Design review of the part built by this model. Coordinates are the model's own, in mm. A direction names the side the tool comes from. Give positions to 0.01 mm unless a question says otherwise; leave off trailing zeros. Order: outer loops, then holes, each group sorted by start corner. A loop starts at its lowest first (then second) coordinate and runs counter-clockwise, first axis right, second up. Notation, with made-up numbers: (32.25, 8.5) -> (74.25, 8.5) arc R21 ccw to (74.25, 13.5) -> close; hole circle Ø2 at (27, 12). An arc over 180 degrees is marked (long way). Return JSON: item names as keys, results as strings.
```python
from build123d import *

# Parameters (mm, degrees)
ESBO_O2_W                  = 2.6
ESBO_O2_H                  = 5.7
CORTE_EXTRUS_O1_DEPTH      = 8
CORTE_EXTRUS_O2_START      = -20
ESBO_O2_2_W                = 2.6
ESBO_O2_2_H                = 5.7
CORTE_EXTRUS_O2_DEPTH      = 8
CORTE_EXTRUS_O3_DEPTH      = 27.223844112
CORTE_EXTRUS_O3_DEPTH_BACK = 27.223844112
ESBO_O3_R                  = 1.65


with BuildPart() as part:
    # Esboço1 → Revolução1 (revolve)
    with BuildSketch(Plane.XY, mode=Mode.PRIVATE) as revolu_o1_sk:
        Polygon((3.05, 20), (10, 20), (10, 0), (2.4, 0), (2.4, 8), (3.05, 8), align=None)
    revolve(revolu_o1_sk.sketch.rotate(Axis((0, 0, 0), (0, 1, 0)), 90), axis=Axis((0, 0, 0), (0, 1, 0)))

    # Esboço2 → Corte-extrusão1 (cut)
    with BuildSketch(Plane(origin=(0, 20, 0), x_dir=(1, 0, 0), z_dir=(0, 1, 0))):
        with Locations((5, 0)):
            Rectangle(ESBO_O2_W, ESBO_O2_H)
        with Locations((-5, 0)):
            Rectangle(ESBO_O2_W, ESBO_O2_H)
    extrude(amount=-CORTE_EXTRUS_O1_DEPTH, mode=Mode.SUBTRACT)

    # Esboço2<2> → Corte-extrusão2 (cut)
    with BuildSketch(Plane(origin=(0, 20, 0), x_dir=(1, 0, 0), z_dir=(0, 1, 0)).offset(CORTE_EXTRUS_O2_START)):
        with Locations((5, 0)):
            Rectangle(ESBO_O2_2_W, ESBO_O2_2_H)
        with Locations((-5, 0)):
            Rectangle(ESBO_O2_2_W, ESBO_O2_2_H)
    extrude(amount=CORTE_EXTRUS_O2_DEPTH, mode=Mode.SUBTRACT)

    # Esboço3 → Corte-extrusão3 (cut, two sides: drawn at the far end of the back side and taken through both)
    with BuildSketch(Plane.ZY.offset(3.7).offset(-CORTE_EXTRUS_O3_DEPTH_BACK)):
        with Locations((0, 4)):
            Circle(ESBO_O3_R)
        with Locations((0, 16)):
            Circle(ESBO_O3_R)
    extrude(amount=CORTE_EXTRUS_O3_DEPTH + CORTE_EXTRUS_O3_DEPTH_BACK, mode=Mode.SUBTRACT)


solid = part.part
```
Item 1: For pin 1 (2 mm diameter, centred on y = 13, z = -3, fed in from -X); pin 2 (3 mm diameter, centred on x = 5, y = 12.5, fed in from -Z); pin 3 (1.3 mm diameter, centred on x = 5, y = 15, fed in from -Z); pin 4 (2.5 mm diameter, centred on y = 4, z = 0, fed in from +X), all flat-tipped, find the tip position at first contact; note any pin that passes through.
Result set:
{"pin 1": "stops at x = -9.8", "pin 2": "stops at z = -9.37", "pin 3": "stops at z = -9", "pin 4": "passes through"}
Item 2: Add section D-D (y = 16). Give the boundary of the cut face in (x, z).
Result set:
{"outline": "(-9.86, -1.65) arc R10 ccw to (9.86, -1.65) -> (6.3, -1.65) -> (6.3, -2.85) -> (3.7, -2.85) -> (3.7, -1.65) -> (2.57, -1.65) arc R3.05 cw to (-2.57, -1.65) -> (-3.7, -1.65) -> (-3.7, -2.85) -> (-6.3, -2.85) -> (-6.3, -1.65) -> close; (-9.86, 1.65) -> (-6.3, 1.65) -> (-6.3, 2.85) -> (-3.7, 2.85) -> (-3.7, 1.65) -> (-2.57, 1.65) arc R3.05 cw to (2.57, 1.65) -> (3.7, 1.65) -> (3.7, 2.85) -> (6.3, 2.85) -> (6.3, 1.65) -> (9.86, 1.65) arc R10 ccw to start"}
Item 3: Add section C-C (x = 8). Give the boundary of the cut face in (y, z), plus the area to 3 significant figures.
Result set:
{"outline": "(0, -6) -> (20, -6) -> (20, 6) -> (0, 6) -> close; hole circle Ø3.3 at (4, 0); hole circle Ø3.3 at (16, 0)", "area": "223 mm^2"}
Item 4: Machinability: for faces 4 (the face through (-5, 16, 2.85)), 5 (the face through (5, 8, 0)), 6 (the face through (8.18, 17.39, 0.89)), which of the approach directions +Z, -Z, +X, -X, +Y, -Y give a long, thin tool a straight path to every point of the face, cutting with its end or side? Answer none if there is none.
Result set:
{"face 4": "+Y", "face 5": "-Y", "face 6": "+X, -X"}
Item 5: Add section A-A (x = 0). Give the boundary of the cut face in (y, z).
Result set:
{"outline": "(0, -10) -> (20, -10) -> (20, -3.05) -> (8, -3.05) -> (8, -2.4) -> (0, -2.4) -> close; (0, 2.4) -> (8, 2.4) -> (8, 3.05) -> (20, 3.05) -> (20, 10) -> (0, 10) -> close"}
Item 6: Mouldability with a two-part tool opening along Z and no side actions: class faces 1 (the face through (2, 0, -2)), 2 (the face through (5, 12, 0)), 3 (the face through (9.76, 9.86, 2.17)) as released by +Z, released by -Z, zero draft, split by the parting line, or undercut.
Result set:
{"face 1": "zero draft", "face 2": "undercut", "face 3": "split by the parting line"}
Item 7: Add section B-B (y = 18.75). Give the boundary of the cut face in (x, z).
Result set:
{"outline": "circle Ø20 at (0, 0); hole (-6.3, -2.85) -> (-3.7, -2.85) -> (-3.7, 2.85) -> (-6.3, 2.85) -> close; hole circle Ø6.1 at (0, 0); hole (3.7, -2.85) -> (6.3, -2.85) -> (6.3, 2.85) -> (3.7, 2.85) -> close"}
Item 8: Wall thickness on L1, parallel to Y at x = 8.75, z = 0; L2, parallel to X at y = 5.5, z = 1.5; L3, parallel to X at y = 6.5, z = -0.5: over which ranges is each line inside the solid? List them lowest first. Write a range as [from, to].
Result set:
{"L1": "y = [0, 2.35], [5.65, 14.35], [17.65, 20]", "L2": "x = [-9.89, -6.3], [-3.7, -1.87], [1.87, 3.7], [6.3, 9.89]", "L3": "x = [-9.99, -6.3], [-3.7, -2.35], [2.35, 3.7], [6.3, 9.99]"}
